Autodesk Inventor part; units mm, degrees
ref_plane "YZ Plane" through (0, 0, 0) normal (1, 0, 0) x (0, 1, 0)
ref_plane "XZ Plane" through (0, 0, 0) normal (0, 1, 0) x (-1, 0, 0)
ref_plane "XY Plane" through (0, 0, 0) normal (0, 0, 1) x (1, 0, 0)
sketch "スケッチ1" plane through (0, 0, 0) normal (0, 0, 1) x (1, 0, 0)
  line L0 (-25, 25) -> (25, 25)
  line L1 (25, 25) -> (25, -25)
  line L2 (25, -25) -> (-25, -25)
  line L3 (-25, -25) -> (-25, 25)
  line L4 (-23, 23) -> (23, 23)
  line L5 (23, 23) -> (23, -23)
  line L6 (23, -23) -> (-23, -23)
  line L7 (-23, -23) -> (-23, 23)
  point P0 (0, 0)
  dimension "d0" = 50
  dimension "d1" = 50
  dimension "d4" = 25
  dimension "d5" = 25
  dimension "d6" = 46
  dimension "d7" = 2
  dimension "d8" = 46
  dimension "d9" = 2
extrude "押し出し1" add sketch "スケッチ1" along normal blind 50
sketch "スケッチ11" plane through (25, -25, 0) normal (1, 0, 0) x (0, 0, -1)
  circle A0 centre (-36.5, 36.5) radius 1.5
  line L0 (-50, 50) -> (-50, 0)
  circle A1 centre (-27.5, 12.5) radius 1.5
  line L1 (0, 50) -> (0, 0)
  line L2 (0, 50) -> (-50, 50)
  point P0 (0, 25)
  point P1 (-50, 43)
  dimension "d109" = 3
  dimension "d128" = 24
  dimension "d237" = 13.5
  dimension "d238" = 27.5
  dimension "d239" = 13.5
hole "穴6" at (25, -12.5, 27.5) at (25, 11.5, 36.5) direction (-1, 0, 0) diameter 4 end through all
sketch "スケッチ16" plane through (-25, -25, 0) normal (-1, 0, 0) x (0, 0, 1)
  line L0 (0, 50) -> (50, 50)
  circle A0 centre (3, 40) radius 1
  circle A1 centre (3, 10) radius 1
  line L1 (0, 48) -> (0, 2)
  line L2 (0, 0) -> (50, 0)
  point P0 (0, 25)
  dimension "d175" = 10
  dimension "d176" = 3
  dimension "d178" = 3
  dimension "d287" = 10
  dimension "d288" = 2
hole "穴16" at (-25, 15, 3) at (-25, -15, 3) direction (1, 0, 0) diameter 2 end through all
sketch "スケッチ15" plane through (-25, -25, 0) normal (0, -1, 0) x (1, 0, 0)
  line L0 (0, 0) -> (0, 50)
  line L1 (50, 0) -> (0, 0)
  circle A0 centre (10, 3) radius 1
  circle A1 centre (40, 3) radius 1
  line L2 (50, 0) -> (50, 50)
  point P0 (49.5, 0)
  point P1 (49.5, 50)
  point P2 (25, 0)
  dimension "d167" = 10
  dimension "d170" = 3
  dimension "d172" = 3
  dimension "d267" = 2
  dimension "d286" = 10
hole "穴17" at (-15, -25, 3) at (15, -25, 3) direction (0, 1, 0) diameter 2 end through all
properties part number "06" material "アルミニウム 6061"
Work out the finished part from the listing and answer in its coordinate system (mm). A direction names the side the tool comes from. Coordinates: 2 decimals unless noted, no trailing zeros. Loops run counter-clockwise (first coordinate to the right, second up) from the corner with the lowest first, then second, coordinate; pieces in that order, holes last.
1) Section A-A (y = -1) is taken. Give the vertices of the cut face in (x, z).
Results:
outline: (-25, 0) - (-23, 0) - (-23, 50) - (-25, 50) - close; (23, 0) - (25, 0) - (25, 50) - (23, 50) - close
2) A flat-ended cylindrical pin translates along its axis: pin 1 (1.6 mm diameter, centred on x = 15, z = 3, fed in from -Y) (3 decimals). Find the tip coordinate at first contact, or state that the pin passes through.
Results:
pin 1: passes through
3) For faces 3 (the flat face through (25, 0, 25)), 4 (the flat face through (23, 0, 25)), determine the directions among +Z, -Z, +X, -X, +Y, -Y from which every point of the face is accessible in a straight line to the end or side of a thin tool.
Results:
face 3: +Z, -Z, +X, +Y, -Y
face 4: +Z, -Z
4) Section B-B (x = -15) is taken. Give the vertices of the cut face in (y, z), plus the area to 3 significant figures.
Results:
outline: (-25, 0) - (-23, 0) - (-23, 2) - (-25, 2) - close; (-25, 4) - (-23, 4) - (-23, 50) - (-25, 50) - close; (23, 0) - (25, 0) - (25, 2) - (23, 2) - close; (23, 4) - (25, 4) - (25, 50) - (23, 50) - close
area: 192 mm2
5) Section C-C (z = 27.5) is taken. Give the vertices of the cut face in (x, y), plus the area to 3 significant figures.
Results:
outline: (-25, -25) - (25, -25) - (25, -14.5) - (23, -14.5) - (23, -23) - (-23, -23) - (-23, -14.5) - (-25, -14.5) - close; (-25, -10.5) - (-23, -10.5) - (-23, 23) - (23, 23) - (23, -10.5) - (25, -10.5) - (25, 25) - (-25, 25) - close
area: 368 mm2
6) For a pull along Z with two mould halves and no side action, classify faces 1 (the cylindrical face through (23.986, -13.101, 25.592)), 2 (the flat face through (-25, 0, 25)) as +Z half, -Z half, draft (parallel to the pull), parting line (faces both ways), or undercut.
Results:
face 1: undercut
face 2: draft
7) Section D-D (y = 11.5) is taken. Give the vertices of the cut face in (x, z), plus the area to 3 significant figures.
Results:
outline: (-25, 0) - (-23, 0) - (-23, 34.5) - (-25, 34.5) - close; (-25, 38.5) - (-23, 38.5) - (-23, 50) - (-25, 50) - close; (23, 0) - (25, 0) - (25, 34.5) - (23, 34.5) - close; (23, 38.5) - (25, 38.5) - (25, 50) - (23, 50) - close
area: 184 mm2
8) Consider probe 1 along Z at (x, y) = (-15, -23.9); probe 2 along Y at (x, z) = (8, 46). Determine where each line is inside the solid, lowest interval first.
Results:
probe 1: z = 0 to 2, 4 to 50
probe 2: y = -25 to -23, 23 to 25
